```python
from build123d import *

# Parameters (mm, degrees)
ESQUISSE1_R             = 6
BOSS_EXTRU_1_DEPTH      = 8
ESQUISSE2_R             = 10.5
ESQUISSE2_R_2           = 1.25
BOSS_EXTRU_2_DEPTH      = 14
ESQUISSE3_R             = 6
BOSS_EXTRU_3_DEPTH      = 2.3
ESQUISSE4_R             = 4
BOSS_EXTRU_4_DEPTH      = 6.25
ESQUISSE5_R             = 3
BOSS_EXTRU_5_DEPTH      = 0.75
ESQUISSE7_R             = 3.5
BOSS_EXTRU_6_DEPTH      = 8
ESQUISSE8_R             = 2.5
BOSS_EXTRU_7_DEPTH      = 0.5
ESQUISSE9_R             = 3
BOSS_EXTRU_8_DEPTH      = 4
ESQUISSE10_R            = 4.75
ENL_V_MAT_EXTRU_1_DEPTH = 21
CHANFREIN1_SIZE         = 0.5
CHANFREIN2_SIZE         = 0.5


with BuildPart() as part:
    # Esquisse1 → Boss.-Extru.1 (new body)
    with BuildSketch(Plane.XY):
        Circle(ESQUISSE1_R)
    extrude(amount=BOSS_EXTRU_1_DEPTH)

    # Esquisse2 → Boss.-Extru.2 (add)
    with BuildSketch(Plane.XY.offset(8)):
        Circle(ESQUISSE2_R)
        with Locations((-7.418567839, -0.026589849)):
            Circle(ESQUISSE2_R_2, mode=Mode.SUBTRACT)
        with Locations((7.418567839, -0.026589849)):
            Circle(ESQUISSE2_R_2, mode=Mode.SUBTRACT)
    extrude(amount=BOSS_EXTRU_2_DEPTH)

    # Esquisse3 → Boss.-Extru.3 (add)
    with BuildSketch(Plane.XY.offset(22)):
        Circle(ESQUISSE3_R)
    extrude(amount=BOSS_EXTRU_3_DEPTH)

    # Esquisse4 → Boss.-Extru.4 (add)
    with BuildSketch(Plane.XY.offset(24.3)):
        Circle(ESQUISSE4_R)
    extrude(amount=BOSS_EXTRU_4_DEPTH)

    # Esquisse5 → Boss.-Extru.5 (add)
    with BuildSketch(Plane.XY.offset(30.55)):
        Circle(ESQUISSE5_R)
    extrude(amount=BOSS_EXTRU_5_DEPTH)

    # Esquisse7 → Boss.-Extru.6 (add)
    with BuildSketch(Plane.XY.offset(31.3)):
        Circle(ESQUISSE7_R)
    extrude(amount=BOSS_EXTRU_6_DEPTH)

    # Esquisse8 → Boss.-Extru.7 (add)
    with BuildSketch(Plane.XY.offset(39.3)):
        Circle(ESQUISSE8_R)
    extrude(amount=BOSS_EXTRU_7_DEPTH)

    # Esquisse9 → Boss.-Extru.8 (add)
    with BuildSketch(Plane.XY.offset(39.8)):
        Circle(ESQUISSE9_R)
    extrude(amount=BOSS_EXTRU_8_DEPTH)

    # Esquisse10 → Enlèv. mat.-Extru.1 (cut)
    with BuildSketch(Plane(origin=(0, 0, 0), x_dir=(-1, 0, 0), z_dir=(0, 0, -1))):
        Circle(ESQUISSE10_R)
    extrude(amount=-ENL_V_MAT_EXTRU_1_DEPTH, mode=Mode.SUBTRACT)

    # Chanfrein1
    chanfrein1_edges = [part.edges().sort_by_distance(p)[0] for p in [
        (-3.5, 0, 39.3),
    ]]
    chamfer(chanfrein1_edges, length=CHANFREIN1_SIZE)

    # Chanfrein2
    chanfrein2_edges = [part.edges().sort_by_distance(p)[0] for p in [
        (-3, 0, 43.8),
    ]]
    chamfer(chanfrein2_edges, length=CHANFREIN2_SIZE)


solid = part.part
```
The model under review builds one solid part; all positions refer to its coordinate system, in mm. A direction names the side the tool comes from. Round coordinates to 2 decimals unless told otherwise and drop trailing zeros. Write each loop counter-clockwise with the first axis right and the second up, starting at its lowest first coordinate (ties: lowest second). Pieces come first, ordered by that corner, then holes. Notation, with made-up numbers: (83.5, -31.75) - (128.5, -31.75) arc R26 ccw to (128.5, 2.25) - close; hole circle Ø10 at (88, 88). An arc over 180 degrees is marked (long way). Answer as CSV lines item,"result". Start each with the question number.
(1) We need section C-C on z = 23.5. State the section outline as (x, y) points.
(2) Draft analysis for pull direction Y (two halves, no side actions). For faces 4 (the cylindrical face through (-2.192, -4.214, 10.353)), 5 (the cylindrical face through (3.233, -1.341, 34.998)), 6 (the flat face through (-2, 2, 39.3)), state which applies: pulls with the +Y half, pulls with the -Y half, needs draft (parallel to the pull), parting line crosses it, or undercut.
(3) We need section A-A on y = -5.5. State the section outline as (x, z) points.
(4) To check wall thickness, follow line 1 (Y direction, x = 0, z = 6.75); line 2 (Y direction, x = 0, z = 11.5); line 3 (Z direction, x = -5, y = -2). State the ranges of each line that lie inside material, in increasing order.
(5) For pin 1 Ø5 at (y, z) = (-5.5, 30.5) entering from +X; pin 2 Ø2 at (x, y) = (-1.5, 1) entering from -Z; pin 3 Ø3 at (x, y) = (-7.42, -0.03) entering from +Z, all flat-tipped, find the tip position at first contact; note any pin that passes through.
(6) For faces 1 (the cylindrical face through (-3, 0, 42)), 2 (the flat face through (0, 0, 21)), 3 (the flat face through (-2, 2, 39.8)), list the 3-axis set-ups (+Z, -Z, +X, -X, +Y, -Y) from which the entire face can be reached by the end or side of a thin tool; tool diameter is ignored.
(7) We need section D-D on z = 28.5. State the section outline as (x, y) points, plus the area to 3 significant figures.
Worked answers:
1,outline,"circle Ø12 at (0, 0)"
2,face 4,"undercut"
2,face 5,"parting line crosses it"
2,face 6,"needs draft"
3,outline,"(-8.94, 8) - (-2.4, 8) - (-2.4, 0) - (2.4, 0) - (2.4, 8) - (8.94, 8) - (8.94, 22) - (2.4, 22) - (2.4, 24.3) - (-2.4, 24.3) - (-2.4, 22) - (-8.94, 22) - close"
4,line 1,"-6 to -4.75, 4.75 to 6"
4,line 2,"-10.5 to -4.75, 4.75 to 10.5"
4,line 3,"0 to 24.3"
5,pin 1,"x = 2.65"
5,pin 2,"z = 21"
5,pin 3,"z = 24.3"
6,face 1,"+Z"
6,face 2,"-Z"
6,face 3,"none"
7,outline,"circle Ø8 at (0, 0)"
7,area,"50.3 mm²"
